from build123d import *

# Parameters (mm, degrees)
SZKIC1_R                         = 14.5
DODANIE_WYCI_GNI_CIE1_DEPTH      = 20
SZKIC2_R                         = 15
DODANIE_WYCI_GNI_CIE2_DEPTH      = 10
ZAOKR_GLENIE1_R                  = 10
SZKIC3_R                         = 5
DODANIE_WYCI_GNI_CIE3_DEPTH      = 28
ZAOKR_GLENIE2_R                  = 0.5
ZAOKR_GLENIE3_R                  = 2
DODANIE_WYCI_GNI_CIE4_REACH      = 74.868
DODANIE_WYCI_GNI_CIE4_END_RADIUS = 14.5
SZKIC4_R                         = 7
SZKIC5_R                         = 5
DODANIE_WYCI_GNI_CIE5_DEPTH      = 35.5


# Some blends are built 0.0001 mm under size
with BuildPart() as part:
    # Szkic1 → Dodanie-wyciągnięcie1 (new body)
    with BuildSketch(Plane.XY):
        Circle(SZKIC1_R)
    extrude(amount=DODANIE_WYCI_GNI_CIE1_DEPTH)

    # Szkic2 → Dodanie-wyciągnięcie2 (add)
    with BuildSketch(Plane.XY.offset(20)):
        Circle(SZKIC2_R)
    extrude(amount=DODANIE_WYCI_GNI_CIE2_DEPTH)

    # Zaokrąglenie1
    zaokr_glenie1_edges = [part.edges().sort_by_distance(p)[0] for p in [
        (-15, 0, 30),
    ]]
    fillet(zaokr_glenie1_edges, radius=ZAOKR_GLENIE1_R - 0.0001)  # a hair under: the kernel refuses the full size

    # Szkic3 → Dodanie-wyciągnięcie3 (add)
    with BuildSketch(Plane.XY.offset(30)):
        Circle(SZKIC3_R)
    extrude(amount=DODANIE_WYCI_GNI_CIE3_DEPTH)

    # Zaokrąglenie2
    # the kernel refuses this fillet: 0.5 mm, written as the material it takes off along each edge
    with BuildSketch(Plane(origin=(0, 0, 20), x_dir=(1, 0, 0), z_dir=(0, -1, 0))) as zaokr_glenie2_piece_1_section:
        with BuildLine():
            CenterArc((14.486838112, 0.5), ZAOKR_GLENIE2_R, 270, 93.01638914)
            Line((14.486838112, 0), (14.486838112, -0.05))
            Line((14.486838112, -0.05), (15, -0.05))
            Line((15, -0.05), (15.05, 0))
            ThreePointArc((15.05, 0), (15.05, 0.0001), (15.0360761, 0.528941884))
            Line((15.0360761, 0.528941884), (14.986145373, 0.526310803))
        make_face()
    zaokr_glenie2_piece_1 = revolve(axis=Axis((0, 0, 20), (0, 0, 1)), mode=Mode.PRIVATE)
    zaokr_glenie2_piece_1 = zaokr_glenie2_piece_1 - Plane(origin=(0, 0, 20.145882789), x_dir=(1, 0, 0), z_dir=(0, 0, -1)) * Cylinder(14.5, 61, mode=Mode.PRIVATE)
    add(zaokr_glenie2_piece_1, mode=Mode.SUBTRACT)

    # Zaokrąglenie3
    zaokr_glenie3_edges = [part.edges().sort_by_distance(p)[0] for p in [
        (-14.5, 0, 0),
    ]]
    fillet(zaokr_glenie3_edges, radius=ZAOKR_GLENIE3_R)

    # Dodanie-wyciągnięcie4: up to this cylinder (the profile starts outside it)
    dodanie_wyci_gni_cie4_end = Plane(origin=(0, 0, 12), z_dir=(0, 0, -1)) * Cylinder(DODANIE_WYCI_GNI_CIE4_END_RADIUS, 179.736, mode=Mode.PRIVATE)
    # Szkic4 → Dodanie-wyciągnięcie4 (add, up to the surface)
    with BuildSketch(Plane(origin=(26.5, 0, 0), x_dir=(0, 0, -1), z_dir=(1, 0, 0)), mode=Mode.PRIVATE) as dodanie_wyci_gni_cie4_sk1:
        with Locations((-12, 0)):
            Circle(SZKIC4_R)
    dodanie_wyci_gni_cie4_tool1 = extrude(dodanie_wyci_gni_cie4_sk1.sketch, amount=-DODANIE_WYCI_GNI_CIE4_REACH, mode=Mode.PRIVATE) - dodanie_wyci_gni_cie4_end
    add(dodanie_wyci_gni_cie4_tool1.solids().sort_by_distance((26.5, 0, 12))[0])

    # Szkic5 → Dodanie-wyciągnięcie5 (add)
    with BuildSketch(Plane(origin=(26.5, 0, 0), x_dir=(0, 0, -1), z_dir=(1, 0, 0))):
        with Locations((-12, 0)):
            Circle(SZKIC5_R)
    extrude(amount=DODANIE_WYCI_GNI_CIE5_DEPTH)


solid = part.part
CAD build for the part. Positions are in the model's coordinates, mm. A direction names the side the tool comes from. Round coordinates to 2 decimals unless told otherwise and drop trailing zeros. Write each loop counter-clockwise with the first axis right and the second up, starting at its lowest first coordinate (ties: lowest second). Pieces come first, ordered by that corner, then holes. Notation, with made-up numbers: M 20.5,-5 L 33.5,-5 A14 cw 33.5,0 Z; hole C 61,-23.5 d10. An arc over 180 degrees is marked long. Put each result on its own line as item: value. Start each with the question number.
1) Drill centre lines: probe 1 along X at (y, z) = (0.25, 50.5); probe 2 along Z at (x, y) = (24, 0.5); probe 3 along Y at (x, z) = (57, 14). Where is each one in solid material? Low to high. Write a range as [from, to].
2) Saw through at A-A, the plane z = 12. Write the cut outline in (x, y), and give its area (3 significant figures).
3) Saw through at C-C, the plane z = 38. Write the cut outline in (x, y).
4) Saw through at B-B, the plane x = 33.5. Write the cut outline in (y, z).
5) 3-axis set-ups, long thin cutter, end or side, ignore diameter. For faces 1 (the cylindrical face through (-1.08, -4.88, 43.8)), 2 (the flat face through (0, 0, 58)), 3 (the cylindrical face through (19.696, 2.103, 5.323)): which of +Z, -Z, +X, -X, +Y, -Y reach the whole face in a straight line?
6) Pin check, flat tips, straight feed: pin 1 Ø5 at (x, z) = (35, 8) entering from -Y; pin 2 Ø3 at (x, y) = (22, 2.5) entering from -Z; pin 3 Ø6 at (x, z) = (52, 9) entering from +Y. Stop position of each tip, or through.
Resolved:
1. probe 1: [-4.99, 4.99]
1. probe 2: [5.02, 18.98]
1. probe 3: [-4.58, 4.58]
2. outline: M 12.7,-7 L 26.5,-7 L 26.5,-5 L 62,-5 L 62,5 L 26.5,5 L 26.5,7 L 12.7,7 A14.5 ccw long Z
2. area: 1,190 mm²
3. outline: C 0,0 d10
4. outline: C 0,12 d10
5. face 1: +Z
5. face 2: +Z, +X, -X, +Y, -Y
5. face 3: +X
6. pin 1: y = -4.77
6. pin 2: z = 5.07
6. pin 3: y = 5
